Design review of the part built by this model. Coordinates are the model's own, in mm. Face numbers are marked on the shaded views. A direction names the side the tool comes from. Give positions to 0.01 mm unless a question says otherwise; leave off trailing zeros. Loops run counter-clockwise (first coordinate to the right, second up) from the corner with the lowest first, then second, coordinate; pieces in that order, holes last.
Autodesk Inventor part; units mm, degrees
ref_plane "YZ Plane" through (0, 0, 0) normal (1, 0, 0) x (0, 1, 0)
ref_plane "XZ Plane" through (0, 0, 0) normal (0, 1, 0) x (-1, 0, 0)
ref_plane "XY Plane" through (0, 0, 0) normal (0, 0, 1) x (1, 0, 0)
sketch "Sketch1" plane through (0, 0, 0) normal (0, 0, 1) x (1, 0, 0)
  line L0 (26.675, -23) -> (-26.675, -23) construction
  line L1 (-26.675, -23) -> (-26.675, 23) construction
  line L2 (-26.675, 23) -> (26.675, 23) construction
  line L3 (26.675, 23) -> (26.675, -23) construction
  line L4 (26.675, -23) -> (-26.675, 23) construction
  line L5 (-26.675, -23) -> (26.675, 23) construction
  line L6 (-26.675, -23) -> (-41.325, -23)
  line L7 (-41.325, -23) -> (-41.325, 15)
  line L8 (-41.325, 15) -> (-26.675, 15)
  line L9 (-26.675, 15) -> (-26.675, -23)
  line L10 (26.675, 23) -> (-11.325, 23)
  line L11 (-11.325, 23) -> (-11.325, 37.65)
  line L12 (-11.325, 37.65) -> (26.675, 37.65)
  line L13 (26.675, 37.65) -> (26.675, 23)
  line L14 (-35.675, -23) -> (-35.675, 32) construction
  line L15 (-35.675, 32) -> (26.675, 32) construction
  circle A0 centre (-35.675, 32) radius 5.65 construction
  line L16 (-26.675, 15) -> (-41.325, 15)
  line L17 (-41.325, 15) -> (-41.325, 37.65)
  line L18 (-35.675, 37.65) -> (-26.675, 37.65)
  line L19 (-26.675, 37.65) -> (-26.675, 15)
  line L20 (-11.325, 23) -> (-41.325, 23)
  line L21 (-41.325, 23) -> (-41.325, 32)
  line L22 (-41.325, 37.65) -> (-11.325, 37.65)
  line L23 (-11.325, 37.65) -> (-11.325, 23)
  arc A1 (-35.675, 37.65) -> (-41.325, 32) centre (-35.675, 32) ccw
  point P0 (0, 0)
  point P1 (0, 0)
  point P2 (-26.675, 23)
  point P3 (-41.325, 32)
  point P4 (-35.675, -14)
  point P5 (-35.675, 6)
  point P6 (17.675, 32)
  point P7 (-2.325, 32)
  dimension "d3" = 9
  dimension "d4" = 9
  dimension "d5" = 5.65
  dimension "d6" = 5.65
  dimension "d8" = 8
  dimension "d9" = 15.35
  dimension "d13" = 5.65
  dimension "d14" = 9
  dimension "d15" = 20
  dimension "d16" = 5.65
  dimension "d17" = 9
  dimension "d18" = 20
  dimension "d33" = 9
  dimension "d35" = 9
extrude "Extrusion1" add sketch "Sketch1" along normal mid plane 6.35 contours L6 L7 L8 L9 | L8 L17 L20 L19 | L20 L17 A1 L18 L19 | L19 L22 L11 L20 | L11 L12 L13 L10
sketch "Sketch2" plane through (0, 0, 3.175) normal (0, 0, 1) x (1, 0, 0)
  line L0 (-41.325, -23) -> (-26.675, -23)
  line L1 (-26.675, -23) -> (-26.675, 23)
  line L2 (-26.675, 23) -> (26.675, 23)
  line L3 (26.675, 23) -> (26.675, 37.65)
  line L4 (26.675, 37.65) -> (-35.675, 37.65)
  arc A0 (-35.675, 37.65) -> (-41.325, 32) centre (-35.675, 32) ccw construction
  line L5 (-41.325, 32) -> (-41.325, -23)
  line L6 (-25.675, 22) -> (-45.675, 22) construction
  line L7 (-45.675, 22) -> (-45.675, 42) construction
  line L8 (-45.675, 42) -> (-25.675, 42) construction
  line L9 (-25.675, 42) -> (-25.675, 22) construction
  line L10 (-25.675, 22) -> (-45.675, 42) construction
  line L11 (-45.675, 22) -> (-25.675, 42) construction
  point P0 (0, 0)
  dimension "d31" = 20
  dimension "d32" = 20
hole "Hole1" at (-35.675, 6, 0) at (-35.675, -14, 0) at (-2.325, 32, 0) at (17.675, 32, 0) at (-35.675, 32, 0) direction (0, 0, -1) diameter 5.3 end through all both
fillet "Fillet1" radius 1 1 edges at (-26.675, 23, 0)
fillet "Fillet2" radius 1 4 edges at (26.675, 23, 0) (26.675, 37.65, 0) (-26.675, -23, 0) (-41.325, -23, 0)
ref_plane "Work Plane1" through (-2.325, 32, 0) normal (0, 1, 0) x (0, 0, 1)
ref_plane "Work Plane2" through (-35.675, 6, 0) normal (1, 0, 0) x (0, 0, 1)
sketch "Sketch3" plane through (0, 0, 3.175) normal (0, 0, 1) x (1, 0, 0)
  arc A0 (-41.325, -22) -> (-40.325, -23) centre (-40.325, -22) ccw
  line L0 (-40.325, -23) -> (-27.675, -23)
  arc A1 (-27.675, -23) -> (-26.675, -22) centre (-27.675, -22) ccw
  line L1 (-26.675, -22) -> (-26.675, 22)
  arc A2 (-25.675, 23) -> (-26.675, 22) centre (-25.675, 22) ccw
  line L2 (-25.675, 23) -> (25.675, 23)
  arc A3 (25.675, 23) -> (26.675, 24) centre (25.675, 24) ccw
  line L3 (26.675, 24) -> (26.675, 36.65)
  arc A4 (26.675, 36.65) -> (25.675, 37.65) centre (25.675, 36.65) ccw
  line L4 (25.675, 37.65) -> (-35.675, 37.65)
  arc A5 (-35.675, 37.65) -> (-41.325, 32) centre (-35.675, 32) ccw
  line L5 (-41.325, 32) -> (-41.325, -22)
  circle A6 centre (-35.675, 32) radius 2.65
  circle A7 centre (17.675, 32) radius 2.65
  circle A8 centre (-2.325, 32) radius 2.65
  circle A9 centre (-35.675, -14) radius 2.65
  circle A10 centre (-35.675, 6) radius 2.65
  point P0 (0, 0)
  point P1 (-17.675, 32)
  point P2 (-35.675, 20.5)
  dimension "d36" = 11.5
  dimension "d37" = 18
hole "Hole2" at (-17.675, 32, 3.175) direction (0, 0, -1) diameter 5.2 end through all
equation "\"d4\" = d3"
equation "\"d6\" = d5"
properties part number "Top Corner Extrusion Plate" material "Aluminum 6061"
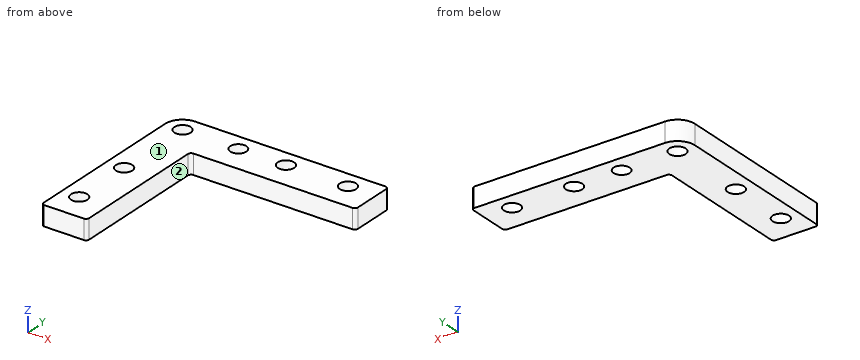
Q1. Take a section at B-B (z = 1.25). Give the boundary of the cut face in (x, y) (3 decimals), plus the area to 3 significant figures.
Results:
outline: (-41.325, -22) arc R1 ccw to (-40.325, -23) - (-27.675, -23) arc R1 ccw to (-26.675, -22) - (-26.675, 22) arc R1 cw to (-25.675, 23) - (25.675, 23) arc R1 ccw to (26.675, 24) - (26.675, 36.65) arc R1 ccw to (25.675, 37.65) - (-35.675, 37.65) arc R5.65 ccw to (-41.325, 32) - close; hole circle Ø5.3 at (-35.675, -14); hole circle Ø5.3 at (-35.675, 6); hole circle Ø5.3 at (-35.675, 32); hole circle Ø5.2 at (-17.675, 32); hole circle Ø5.3 at (-2.325, 32); hole circle Ø5.3 at (17.675, 32)
area: 1,530 mm2
Q2. Take a section at D-D (x = 8). Give the boundary of the cut face in (y, z) (3 decimals), plus the area to 3 significant figures.
Results:
outline: (23, -3.175) - (37.65, -3.175) - (37.65, 3.175) - (23, 3.175) - close
area: 93.0 mm2
Q3. Insertion check: pin 1 (4.5 mm diameter, centred on x = -17.675, y = 32, fed in from -Z); pin 2 (1.5 mm diameter, centred on y = -5, z = 1.5, fed in from +X) (3 decimals). Each pin has a flat end and moves straight along its axis. Give the tip position at first contact, or say it passes through.
Results:
pin 1: passes through
pin 2: stops at x = -26.675
Q4. Wall thickness on line 1 (X direction, y = -14, z = -1.5) (3 decimals); line 2 (X direction, y = 32, z = -1) (3 decimals); line 3 (Y direction, x = 17.5, z = 1): over which ranges is each line inside the solid? List them lowest first.
Results:
line 1: x = -41.325 to -38.325, -33.025 to -26.675
line 2: x = -41.325 to -38.325, -33.025 to -20.275, -15.075 to -4.975, 0.325 to 15.025, 20.325 to 26.675
line 3: y = 23 to 29.36, 34.64 to 37.65
Q5. Take a section at C-C (y = -10). Give the boundary of the cut face in (x, z) (3 decimals), plus the area to 3 significant figures.
Results:
outline: (-41.325, -3.175) - (-26.675, -3.175) - (-26.675, 3.175) - (-41.325, 3.175) - close
area: 93.0 mm2
Q6. Take a section at A-A (y = 6). Give the boundary of the cut face in (x, z) (3 decimals), plus the area to 3 significant figures.
Results:
outline: (-41.325, -3.175) - (-38.325, -3.175) - (-38.325, 3.175) - (-41.325, 3.175) - close; (-33.025, -3.175) - (-26.675, -3.175) - (-26.675, 3.175) - (-33.025, 3.175) - close
area: 59.4 mm2
Q7. Tool access review of the marked faces 1 and 2: name each direction out of +Z, -Z, +X, -X, +Y, -Y from which nothing blocks a thin tool from reaching the whole face with its end or side.
Results:
face 1: +Z, +X, -X, +Y, -Y
face 2: +Z, -Z, +X, -Y
